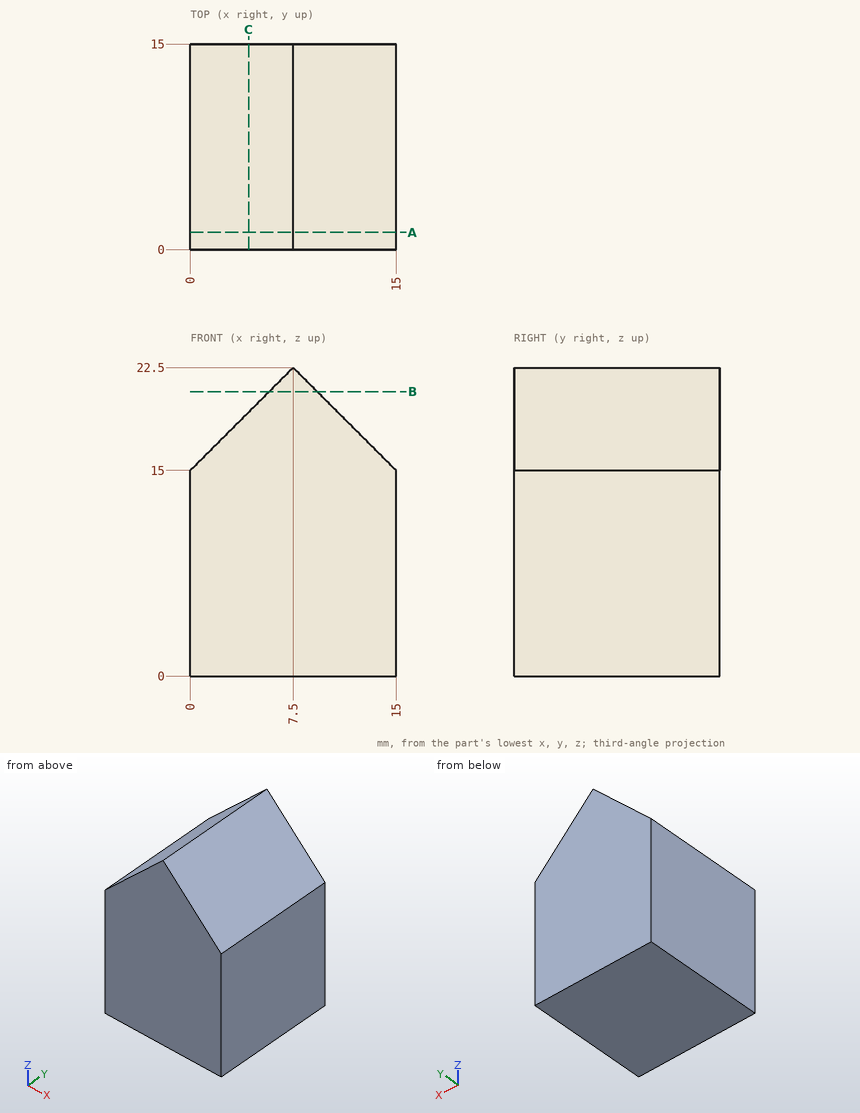
Here's the drawing with two shaded views (mm, measured from the low corner). I have some questions. Coordinates: 2 decimals unless noted, no trailing zeros. Write each loop counter-clockwise with the first axis right and the second up, starting at its lowest first coordinate (ties: lowest second). Pieces come first, ordered by that corner, then holes. Notation, with made-up numbers: (86, -31) -> (96, -31) arc R20 cw to (96, -11) -> close; hole circle Ø2 at (-31, 54.5). An arc over 180 degrees is marked (long way). Use a Markdown table: item, result. Add a question column.
(1) Please list where these lines run through material, in increasing order: line 1 (Z direction, x = 12.25, y = 1); line 2 (Z direction, x = 6, y = 12); line 3 (X direction, y = 6.5, z = 19.5).
(2) If we section it at B-B, the plane z = 20.75: Write out the boundary of the cut face in (x, y).
(3) I'm going to push flat-ended pins straight in: P1, Ø8, axis at x = 13, y = 4.5, coming from the +Z side; P2, Ø6, axis at x = 3, y = 6.5, coming from the -Z side; P3, Ø2, axis at y = 12, z = 19, coming from the +X side. Where does each tip first touch, or does it pass through?
(4) If we section it at C-C, the plane x = 4.25: Write out the boundary of the cut face in (y, z), and give its area (3 significant figures).
(5) If we section it at A-A, the plane y = 1.25: Write out the boundary of the cut face in (x, z), and give its area (3 significant figures).
Outcome:
| question | item | result |
|---|---|---|
| 1 | line 1 | z = 0 to 17.75 |
| 1 | line 2 | z = 0 to 21 |
| 1 | line 3 | x = 4.5 to 10.5 |
| 2 | outline | (5.75, 0) -> (9.25, 0) -> (9.25, 15) -> (5.75, 15) -> close |
| 3 | P1 | stops at z = 21 |
| 3 | P2 | stops at z = 0 |
| 3 | P3 | stops at x = 12 |
| 4 | outline | (0, 0) -> (15, 0) -> (15, 19.25) -> (0, 19.25) -> close |
| 4 | area | 289 mm^2 |
| 5 | outline | (0, 0) -> (15, 0) -> (15, 15) -> (7.5, 22.5) -> (0, 15) -> close |
| 5 | area | 281 mm^2 |
